from build123d import *

# Parameters (mm, degrees)
F0_W     = 6
F0_H     = 16
F0_R     = 1.4
F1_DEPTH = 6.4
F2_R     = 2.99999
F3_W     = 1.9810468791
F3_H     = 4.4
F3_W_2   = 8
F3_H_2   = 3
F4_DEPTH = 8


# Not quite as in the source:
# - a fillet or chamfer is up to 0.001 mm smaller than in the source, because OpenCascade refuses the exact size


with BuildPart() as f1:
    # F0 (on Top) → F1 (new body)
    with BuildSketch(Plane.XY):
        Rectangle(F0_W, F0_H)
        with Locations((0, 5)):
            Circle(F0_R, mode=Mode.SUBTRACT)
    extrude(amount=F1_DEPTH)

    # F2 (radius 3 in the source; OpenCascade refuses exactly that, so slightly less here)
    f2_edges = [f1.edges().sort_by_distance(p)[0] for p in [
        (3, 8, 3.2),
        (-3, 8, 3.2),
    ]]
    fillet(f2_edges, radius=F2_R)

    # F3 (on face) → F4 (cut)
    with BuildSketch(Plane.YZ.offset(3)):
        Polygon((5.00001, 6.4), (5.00001, 2), (8.0189631209, 2), (8.0189631209, 7), (3.0189631209, 7), (3.0189631209, 6.4), align=None)
        with Locations((4.0094865604, 4.2)):
            Rectangle(F3_W, F3_H)
        with Locations((-1.9810368791, 1.5)):
            Rectangle(F3_W_2, F3_H_2)
    extrude(amount=-F4_DEPTH, mode=Mode.SUBTRACT)


solid = f1.part
Could you check a few things on this model? Use its own coordinates, in mm. A direction names the side the tool comes from. Give positions to 0.01 mm unless a question says otherwise; leave off trailing zeros. Order: outer loops, then holes, each group sorted by start corner. A loop starts at its lowest first (then second) coordinate and runs counter-clockwise, first axis right, second up. Notation, with made-up numbers: (23, -20) - (72, -20) arc R15 cw to (72, -1) - close; hole circle Ø9 at (44.5, 40.25). An arc over 180 degrees is marked (long way). One line per item, written item: value. Start each with the question number.
1. For faces 5 (the face through (-2.14, 7.1, 1.01)), 6 (the face through (0, -2, 3)), which set-ups out of +Z, -Z, +X, -X, +Y, -Y let a thin tool reach every point of the face, with its end or its side?
2. Imagine slicing it at D-D on x = -1.75. List the corners of the cut face in (y, z) for me, plus the area to 3 significant figures.
3. Imagine slicing it at C-C on x = -1. List the corners of the cut face in (y, z) for me, plus the area to 3 significant figures.
4. If I drill on probe 1 along Y at (x, z) = (0, 1.45); probe 2 along X at (y, z) = (5, 0.9); probe 3 along Z at (x, y) = (0.5, -4.25), over which ranges is the centre line in solid material (lowest first)?
5. Imagine slicing it at B-B on y = 6. List the corners of the cut face in (x, z) for me, plus the area to 3 significant figures.
6. Thinking about a two-plate mould opening in Y: for faces 1 (the face through (0, -8, 3)), 2 (the face through (0, 3.019, 4)), 3 (the face through (-1.03, 5.95, 0.99)), 4 (the face through (0, 7, 2)), which applies, +Y half, -Y half, draft (parallel to the pull), parting line (faces both ways), or undercut?
7. Imagine slicing it at A-A on z = 1.75. Give the number of separate pieces and of enclosed holes in the cut face, plus the area to 3 significant figures.
8. For P1, Ø1, axis at x = -1.5, y = 4, coming from the +Z side; P2, Ø2, axis at x = -0.5, z = 4, coming from the +Y side; P3, Ø0.9, axis at x = 1, z = 1, coming from the +Y side; P4, Ø2, axis at x = 0, y = 5, coming from the +Z side, each with a flat end and sliding along its axis, tell me the tip position at first contact or that it passes through.
Values:
1. face 5: +Z, -Z, -X, +Y
1. face 6: -Z, +X, -X
2. outline: (-8, 0) - (-5.98, 0) - (-5.98, 3) - (2.02, 3) - (2.02, 0) - (7.44, 0) - (7.44, 2) - (3.02, 2) - (3.02, 6.4) - (-8, 6.4) - close
2. area: 55.4 mm²
3. outline: (-8, 0) - (-5.98, 0) - (-5.98, 3) - (2.02, 3) - (2.02, 0) - (4.02, 0) - (4.02, 2) - (3.02, 2) - (3.02, 6.4) - (-8, 6.4) - close; (5.98, 0) - (7.83, 0) - (7.83, 2) - (5.98, 2) - close
3. area: 52.2 mm²
4. probe 1: -8 to -5.98, 2.02 to 3.6, 6.4 to 8
4. probe 2: -3 to -1.4, 1.4 to 3
4. probe 3: 3 to 6.4
5. outline: (-2.83, 0) - (-0.98, 0) - (-0.98, 2) - (-2.83, 2) - close; (0.98, 0) - (2.83, 0) - (2.83, 2) - (0.98, 2) - close
5. area: 7.39 mm²
6. face 1: -Y half
6. face 2: +Y half
6. face 3: undercut
6. face 4: draft
7. separate pieces: 2
7. enclosed holes: 1
7. area: 38.0 mm²
8. P1: z = 2
8. P2: y = 3.02
8. P3: y = 7.95
8. P4: through
